Verification items for the finished model (mm, model axes). Face numbers are marked on the shaded views. Round coordinates to 2 decimals unless told otherwise and drop trailing zeros. Write each loop counter-clockwise with the first axis right and the second up, starting at its lowest first coordinate (ties: lowest second). Pieces come first, ordered by that corner, then holes. Notation, with made-up numbers: (63.25, 37) - (112.25, 37) arc R7 ccw to (112.25, 44) - close; hole circle Ø4 at (47.5, 3.25). An arc over 180 degrees is marked (long way). Answer as a JSON object with one key per item and string values.
```python
from build123d import *

# Parameters (mm, degrees)
SKETCH1_R           = 6.25
BOSS_EXTRUDE1_DEPTH = 50
SKETCH2_R           = 4.5
CUT_EXTRUDE1_DEPTH  = 1
SKETCH3_W           = 3.8
SKETCH3_H           = 3.8
BOSS_EXTRUDE2_DEPTH = 5


with BuildPart() as part:
    # Sketch1 → Boss-Extrude1 (new body)
    with BuildSketch(Plane(origin=(0, 0, 0), x_dir=(1, 0, 0), z_dir=(0, 1, 0))):
        Circle(SKETCH1_R)
    extrude(amount=BOSS_EXTRUDE1_DEPTH)

    # Sketch2 → Cut-Extrude1 (cut)
    with BuildSketch(Plane.XZ):
        Circle(SKETCH2_R)
    extrude(amount=-CUT_EXTRUDE1_DEPTH, mode=Mode.SUBTRACT)

    # Sketch3 → Boss-Extrude2 (add)
    with BuildSketch(Plane(origin=(0, 1, 0), x_dir=(-1, 0, 0), z_dir=(0, -1, 0))):
        Rectangle(SKETCH3_W, SKETCH3_H)
    extrude(amount=BOSS_EXTRUDE2_DEPTH)


solid = part.part
```
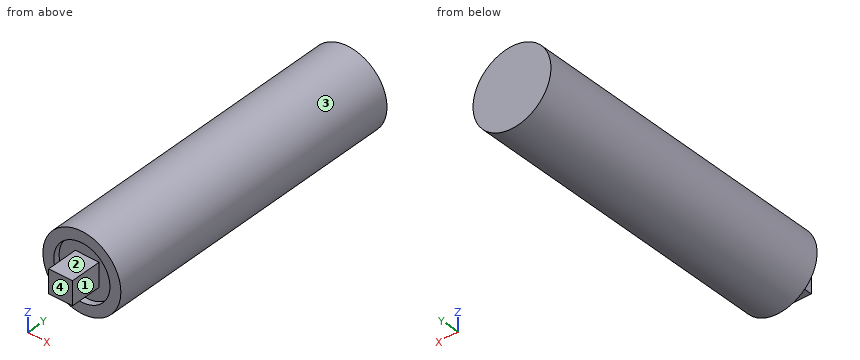
1. Material ranges on probe 1 along Z at (x, y) = (0, 0.8); probe 2 along Y at (x, z) = (5, 0.75); probe 3 along Y at (x, z) = (2.25, 2.25), recorded low to high. Write a range as from..to.
Completed:
{"probe 1": "z = -6.25..-4.5, -1.9..1.9, 4.5..6.25", "probe 2": "y = 0..50", "probe 3": "y = 1..50"}
2. Go/stop test with flat-tipped pins: pin 1 (2 mm diameter, centred on y = 22.5, z = 3.5, fed in from +X); pin 2 (4 mm diameter, centred on x = -3, z = -4.5, fed in from -Y); pin 3 (5 mm diameter, centred on x = -5, y = 13, fed in from -Z). Record where each tip stops, or that it passes through.
Completed:
{"pin 1": "stops at x = 5.73", "pin 2": "stops at y = 0", "pin 3": "stops at z = -5.73"}
3. Cross-section at A-A (x = 0). Record the boundary of the cut face in (y, z), plus the area to 3 significant figures.
Completed:
{"outline": "(-4, -1.9) - (1, -1.9) - (1, -4.5) - (0, -4.5) - (0, -6.25) - (50, -6.25) - (50, 6.25) - (0, 6.25) - (0, 4.5) - (1, 4.5) - (1, 1.9) - (-4, 1.9) - close", "area": "635 mm^2"}
4. Mould release check, pull along Z, two halves, no side actions. Record for the marked faces 1, 2, 3 and 4: released by +Z, released by -Z, zero draft, split by the parting line, or undercut.
Completed:
{"face 1": "undercut", "face 2": "undercut", "face 3": "split by the parting line", "face 4": "zero draft"}
5. Cross-section at B-B (z = 0). Record the boundary of the cut face in (x, y).
Completed:
{"outline": "(-6.25, 0) - (-4.5, 0) - (-4.5, 1) - (-1.9, 1) - (-1.9, -4) - (1.9, -4) - (1.9, 1) - (4.5, 1) - (4.5, 0) - (6.25, 0) - (6.25, 50) - (-6.25, 50) - close"}
6. Cross-section at C-C (y = 44). Record the boundary of the cut face in (x, z), plus the area to 3 significant figures.
Completed:
{"outline": "circle Ø12.5 at (0, 0)", "area": "123 mm^2"}
7. Cross-section at D-D (z = 3.5). Record the boundary of the cut face in (x, y), plus the area to 3 significant figures.
Completed:
{"outline": "(-5.18, 0) - (-2.83, 0) - (-2.83, 1) - (2.83, 1) - (2.83, 0) - (5.18, 0) - (5.18, 50) - (-5.18, 50) - close", "area": "512 mm^2"}
